CAD build for the part. Positions are in the model's coordinates, mm. Face numbers are marked on the shaded views. A direction names the side the tool comes from. Coordinates: 2 decimals unless noted, no trailing zeros. Loops run counter-clockwise (first coordinate to the right, second up) from the corner with the lowest first, then second, coordinate; pieces in that order, holes last. Notation, with made-up numbers: (-34.75, 79.25) -> (-24.75, 79.25) arc R26 ccw to (-24.75, 102.25) -> close; hole circle Ø9 at (18.25, 83.5). An arc over 180 degrees is marked (long way). Return JSON: item names as keys, results as strings. Group by question number.
(1) Saw through at C-C on y = 1.85. Write the cut outline in (x, z), then the cut area to 3 significant figures.
(2) Saw through at B-B on z = 1.25. Write the cut outline in (x, y).
(3) Flat gauge pins, fed straight in: pin 1 Ø1.6 at (y, z) = (2, 1.5) entering from +X; pin 2 Ø1.5 at (x, z) = (3.5, 3) entering from +Y; pin 3 Ø1.6 at (y, z) = (1.5, 3.75) entering from +X. Where does each tip first touch, or does it go through?
(4) Saw through at A-A on x = 0. Write the cut outline in (y, z), then the cut area to 3 significant figures.
(5) Tool access for the marked faces 1, 2 and 3: list every direction of +Z, -Z, +X, -X, +Y, -Y with a clear straight run to the whole face (end or side of a thin tool).
(6) Probe L1, parallel to Y at x = 10.3, z = 1.25; L2, parallel to Z at x = 3.25, y = 0.7; L3, parallel to Y at x = 5.5, z = 3.1. List the from-to ranges inside material, lowest first.
(7) Saw through at D-D on y = 0.7. Write the cut outline in (x, z).
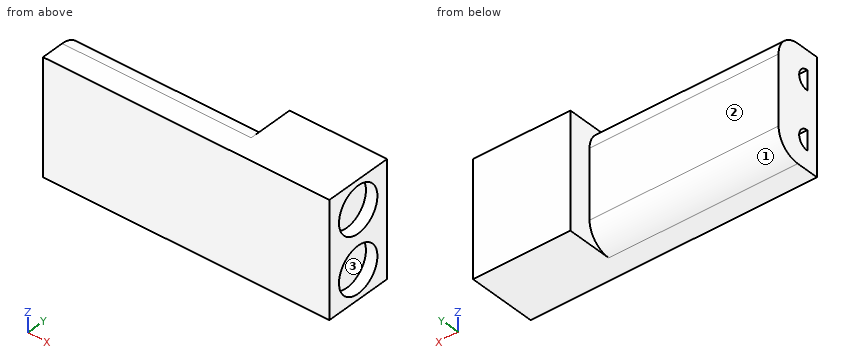
```python
from build123d import *

# Parameters (mm, degrees)
BOSS_EXTRUDE1_DEPTH = 5
FILLET4_R           = 1
CUT_EXTRUDE3_DEPTH  = 10
SKETCH5_R           = 1
CUT_EXTRUDE4_DEPTH  = 0.5


with BuildPart() as part:
    # Sketch1 → Boss-Extrude1 (new body)
    with BuildSketch(Plane.XY):
        Polygon((10.416666667, 3), (10.416666667, 0), (-2.083333333, 0), (-2.083333333, 2), (6.166666667, 2), (6.166666667, 3), align=None)
    extrude(amount=BOSS_EXTRUDE1_DEPTH)

    # Fillet4
    fillet4_edges = [part.edges().sort_by_distance(p)[0] for p in [
        (2.041666667, 2, 5),
        (2.041666667, 2, 0),
    ]]
    fillet(fillet4_edges, radius=FILLET4_R)

    # Sketch2 → Cut-Extrude3 (cut)
    with BuildSketch(Plane.ZY.offset(2.083333333)):
        with BuildLine():
            Line((4.177757267, 0.5), (3.322242733, 0.5))
            ThreePointArc((3.322242733, 0.5), (3.75, 0.927757267), (4.177757267, 0.5))
        make_face()
        with BuildLine():
            Line((0.822242733, 0.5), (1.677757267, 0.5))
            ThreePointArc((1.677757267, 0.5), (1.25, 0.927757267), (0.822242733, 0.5))
        make_face()
    extrude(amount=-CUT_EXTRUDE3_DEPTH, mode=Mode.SUBTRACT)

    # Sketch5 → Cut-Extrude4 (cut)
    with BuildSketch(Plane(origin=(10.416666667, 0, 0), x_dir=(0, 0, -1), z_dir=(1, 0, 0))):
        with Locations((-3.75, 1.5)):
            Circle(SKETCH5_R)
        with Locations(Location((-1.25, 1.5, 0), (0, 0, 180))):
            Circle(SKETCH5_R)
    extrude(amount=-CUT_EXTRUDE4_DEPTH, mode=Mode.SUBTRACT)


solid = part.part
```
Geometry results:
{
 "1": {"outline": "(-2.08, 0.47) -> (6.17, 0.47) -> (6.17, 0) -> (10.42, 0) -> (10.42, 0.31) -> (9.92, 0.31) -> (9.92, 2.19) -> (10.42, 2.19) -> (10.42, 2.81) -> (9.92, 2.81) -> (9.92, 4.69) -> (10.42, 4.69) -> (10.42, 5) -> (6.17, 5) -> (6.17, 4.53) -> (-2.08, 4.53) -> close", "area": "52.8 mm²"},
 "2": {"outline": "(-2.08, 0) -> (10.42, 0) -> (10.42, 0.5) -> (9.92, 0.5) -> (9.92, 2.5) -> (10.42, 2.5) -> (10.42, 3) -> (6.17, 3) -> (6.17, 2) -> (-2.08, 2) -> (-2.08, 0.93) -> (7.92, 0.93) -> (7.92, 0.5) -> (-2.08, 0.5) -> close"},
 "3": {"pin 1": "x = 10.42", "pin 2": "y = 2", "pin 3": "x = 9.92"},
 "4": {"outline": "(0, 0) -> (1, 0) arc R1 ccw to (2, 1) -> (2, 4) arc R1 ccw to (1, 5) -> (0, 5) -> close; hole (0.5, 0.82) arc R0.43 ccw to (0.5, 1.68) -> close; hole (0.5, 3.32) arc R0.43 ccw to (0.5, 4.18) -> close", "area": "9.00 mm²"},
 "5": {"face 1": "-Z, -X, +Y", "face 2": "+Z, -Z, -X, +Y", "face 3": "+X"},
 "6": {"L1": "0 to 0.5, 2.5 to 3", "L2": "0 to 0.87, 1.63 to 3.37, 4.13 to 5", "L3": "0 to 2"},
 "7": {"outline": "(-2.08, 0) -> (10.42, 0) -> (10.42, 0.65) -> (9.92, 0.65) -> (9.92, 1.85) -> (10.42, 1.85) -> (10.42, 3.15) -> (9.92, 3.15) -> (9.92, 4.35) -> (10.42, 4.35) -> (10.42, 5) -> (-2.08, 5) -> (-2.08, 4.13) -> (7.92, 4.13) -> (7.92, 3.37) -> (-2.08, 3.37) -> (-2.08, 1.63) -> (7.92, 1.63) -> (7.92, 0.87) -> (-2.08, 0.87) -> close"}
}
